```python
from build123d import *

# Parameters (mm, degrees)
SKETCH1_R           = 11.049
BOSS_EXTRUDE1_DEPTH = 25.4
SKETCH2_R           = 15.875
BOSS_EXTRUDE2_DEPTH = 6.35
SKETCH3_R           = 5.5
CUT_EXTRUDE1_DEPTH  = 39.885649667
CHAMFER1_SIZE       = 0.299999908


with BuildPart() as part:
    # Sketch1 → Boss-Extrude1 (new body)
    with BuildSketch(Plane(origin=(0, 0, 0), x_dir=(1, 0, 0), z_dir=(0, 1, 0))):
        with Locations(Location((0, 0, 0), (0, 0, 270))):
            Circle(SKETCH1_R)
    extrude(amount=BOSS_EXTRUDE1_DEPTH)

    # Sketch2 → Boss-Extrude2 (add)
    with BuildSketch(Plane.XZ):
        with Locations(Location((0, 0, 0), (0, 0, 270))):
            Circle(SKETCH2_R)
    extrude(amount=BOSS_EXTRUDE2_DEPTH)

    # Sketch3 → Cut-Extrude1 (cut, through all)
    with BuildSketch(Plane.XZ.offset(6.35)):
        with Locations(Location((0, 0, 0), (0, 0, 270))):
            Circle(SKETCH3_R)
    extrude(amount=-CUT_EXTRUDE1_DEPTH, mode=Mode.SUBTRACT)

    # Chamfer1
    chamfer1_edges = [part.edges().sort_by_distance(p)[0] for p in [
        (0, 25.4, 5.5),
        (0, -6.35, 5.5),
        (0, 25.4, -11.049),
        (0, 0, 15.875),
        (0, -6.35, 15.875),
    ]]
    chamfer(chamfer1_edges, length=CHAMFER1_SIZE)


solid = part.part
```
Verification items for the finished model (mm, model axes). A direction names the side the tool comes from. Coordinates: 2 decimals unless noted, no trailing zeros. Order: outer loops, then holes, each group sorted by start corner. A loop starts at its lowest first (then second) coordinate and runs counter-clockwise, first axis right, second up. Notation, with made-up numbers: (-6, 78) - (32, 78) arc R22 cw to (32, 96) - close; hole circle Ø1 at (-4, 87). An arc over 180 degrees is marked (long way). Return JSON: item names as keys, results as strings.
(1) Go/stop test with flat-tipped pins: pin 1 (12 mm diameter, centred on y = 6.5, z = 3.5, fed in from -X); pin 2 (2 mm diameter, centred on y = 1.5, z = 3, fed in from +X); pin 3 (12 mm diameter, centred on x = 3.5, y = 18, fed in from -Z). Record where each tip stops, or that it passes through.
Filled sheet:
{"pin 1": "stops at x = -11.05", "pin 2": "stops at x = 10.87", "pin 3": "stops at z = -11.05"}
(2) Access from +Z, -Z, +X, -X, +Y, -Y to the whole of each face (thin tool, end or side, straight path). Record for faces 4 (the flat face through (11, 0, -3)), 5 (the cylindrical face through (-15.497, -3.135, 3.441)).
Filled sheet:
{"face 4": "+Y", "face 5": "+Y, -Y"}
(3) Thickness scan on line 1 along X through (y, z) = (15, 0); line 2 along Y through (x, z) = (-12, -2); line 3 along Z through (x, y) = (4.5, 21). Record the ranges inside material, lowest first.
Filled sheet:
{"line 1": "x = -11.05 to -5.5, 5.5 to 11.05", "line 2": "y = -6.35 to 0", "line 3": "z = -10.09 to -3.16, 3.16 to 10.09"}
(4) Section check A-A, the plane z = 0. Record the cut outline in (x, y) (3 decimals).
Filled sheet:
{"outline": "(-15.875, -6.05) - (-15.575, -6.35) - (-5.8, -6.35) - (-5.5, -6.05) - (-5.5, 25.1) - (-5.8, 25.4) - (-10.749, 25.4) - (-11.049, 25.1) - (-11.049, 0) - (-15.575, 0) - (-15.875, -0.3) - close; (5.5, -6.05) - (5.8, -6.35) - (15.575, -6.35) - (15.875, -6.05) - (15.875, -0.3) - (15.575, 0) - (11.049, 0) - (11.049, 25.1) - (10.749, 25.4) - (5.8, 25.4) - (5.5, 25.1) - close"}
(5) Section check B-B, the plane x = 0. Record the cut outline in (y, z) (3 decimals), and give its area (3 significant figures).
Filled sheet:
{"outline": "(-6.35, -15.575) - (-6.05, -15.875) - (-0.3, -15.875) - (0, -15.575) - (0, -11.049) - (25.1, -11.049) - (25.4, -10.749) - (25.4, -5.8) - (25.1, -5.5) - (-6.05, -5.5) - (-6.35, -5.8) - close; (-6.35, 5.8) - (-6.05, 5.5) - (25.1, 5.5) - (25.4, 5.8) - (25.4, 10.749) - (25.1, 11.049) - (0, 11.049) - (0, 15.575) - (-0.3, 15.875) - (-6.05, 15.875) - (-6.35, 15.575) - close", "area": "413 mm^2"}
(6) Section check C-C, the plane y = 7. Record the cut outline in (x, z).
Filled sheet:
{"outline": "circle Ø22.1 at (0, 0); hole circle Ø11 at (0, 0)"}
(7) Mould release check, pull along Z, two halves, no side actions. Record for faces 1 (the cylindrical face through (-5.37, 9.31, 1.19)), 2 (the flat face through (-5, 25.4, 5)), 3 (the cylindrical face through (7.47, 12.37, -8.14)): pulls with the +Z half, pulls with the -Z half, needs draft (parallel to the pull), parting line crosses it, or undercut.
Filled sheet:
{"face 1": "undercut", "face 2": "needs draft", "face 3": "parting line crosses it"}
